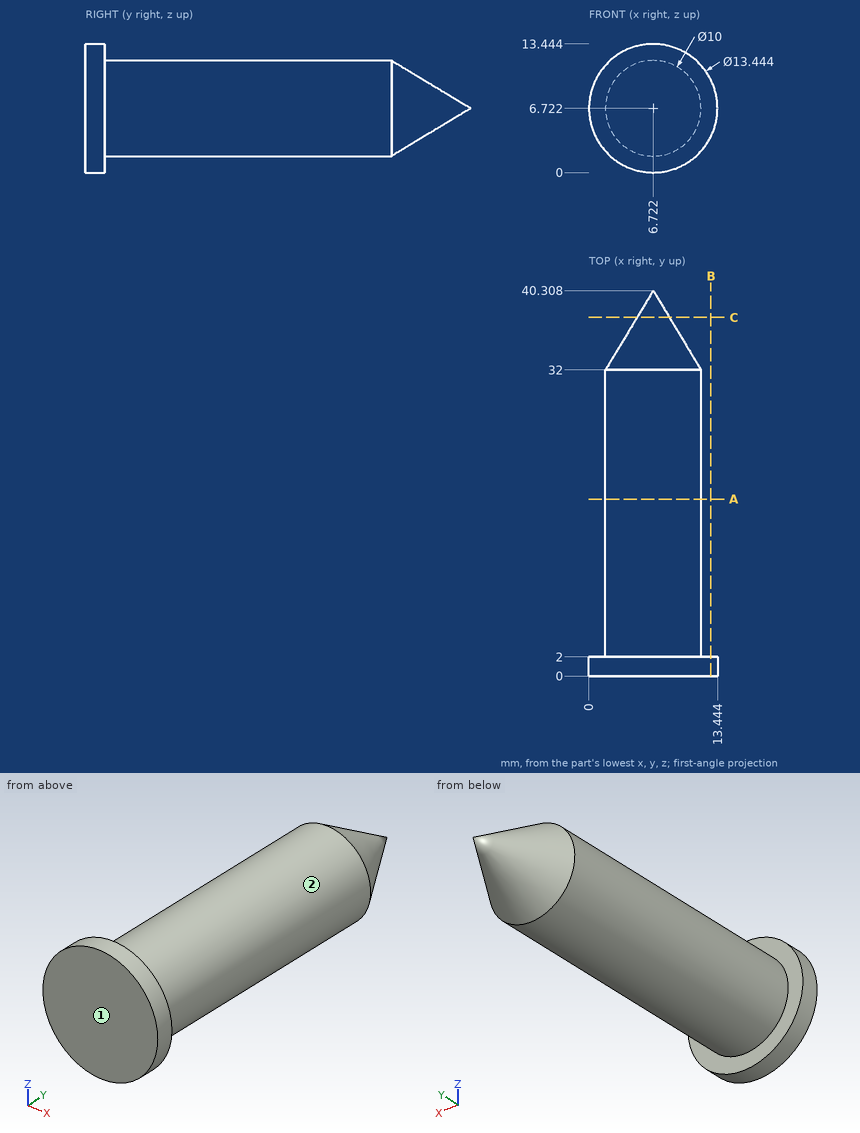
Here's the drawing with two shaded views (mm, measured from the low corner). I have some questions. A direction names the side the tool comes from. Round coordinates to 2 decimals unless told otherwise and drop trailing zeros. Write each loop counter-clockwise with the first axis right and the second up, starting at its lowest first coordinate (ties: lowest second). Pieces come first, ordered by that corner, then holes. Notation, with made-up numbers: M 80,7 L 113,7 A17 cw 113,16 Z; hole C 7,24 d7. An arc over 180 degrees is marked long. Answer in a Markdown table with one row per item. Add a question column.
Q1. Imagine slicing it at A-A (y = 18.5). Please give me the cut outline in (x, z).
Q2. On a 3-axis mill with a long thin cutter (end or side, diameter ignored), from which of +Z, -Z, +X, -X, +Y, -Y can I reach the whole of each face in a straight line? I mean the marked faces 1 and 2. Say none if no direction works.
Q3. Will these pins go through, and if not, where does the flat tip stop? pin 1 Ø4 at (y, z) = (14, 3) entering from +X (1 decimal); pin 2 Ø1 at (x, y) = (6, 7.5) entering from -Z; pin 3 Ø2 at (y, z) = (23.5, 7.5) entering from +X.
Q4. If I drill on line 1 (Y direction, x = 12.25, z = 4.25); line 2 (Y direction, x = 3.75, z = 3) (1 decimal); line 3 (X direction, y = 11, z = 5.75), over which ranges is the centre line in solid material (lowest first)? Write a range as from..to.
Q5. Imagine slicing it at C-C (y = 37.5). Please give me the cut outline in (x, z).
Q6. Imagine slicing it at B-B (x = 12.75). Please give me the cut outline in (y, z) (1 decimal), then the cut area to 3 significant figures.
Values:
| question | item | result |
|---|---|---|
| 1 | outline | C 6.72,6.72 d10 |
| 2 | face 1 | +Z, -Z, +X, -X, -Y |
| 2 | face 2 | +Y |
| 3 | pin 1 | x = 11.4 |
| 3 | pin 2 | z = 1.73 |
| 3 | pin 3 | x = 11.72 |
| 4 | line 1 | 0..2 |
| 4 | line 2 | 0..32.4 |
| 4 | line 3 | 1.82..11.63 |
| 5 | outline | C 6.72,6.72 d3.38 |
| 6 | outline | M 0,3.7 L 2,3.7 L 2,9.7 L 0,9.7 Z |
| 6 | area | 11.9 mm^2 |
